For this review, take the finished solid that the model builds, in its own axes (mm). Face numbers are marked on the shaded views. Give positions to 0.01 mm unless a question says otherwise; leave off trailing zeros. Write each loop counter-clockwise with the first axis right and the second up, starting at its lowest first coordinate (ties: lowest second). Pieces come first, ordered by that corner, then holes.
Q1. We need section C-C (y = -45.5). Write out the cut boundary in (x, z), then the cut area to 3 significant figures.
Q2. We need section A-A (y = 6). Write out the cut boundary in (x, z).
Q3. We need section D-D (x = -46). Write out the cut boundary in (y, z), then the cut area to 3 significant figures.
Q4. Insertion check: P1, Ø1.5, axis at x = 0.5, y = -30, coming from the -Z side; P2, Ø12, axis at x = 58.5, y = -37.5, coming from the +Z side; P3, Ø4, axis at x = -30, y = 0, coming from the -Z side. Each pin has a flat end and moves straight along its axis. Give the tip position at first contact, or say it passes through.
Q5. Mouldability with a two-part tool opening along X and no side actions: class the marked faces 1, 2 and 3 as released by +X, released by -X, zero draft, split by the parting line, or undercut.
Q6. For line 1 (Y direction, x = 0, z = 0.5); line 2 (Z direction, x = -37.5, y = 56); line 3 (X direction, y = 0, z = -1.5), list the stretches that pass through material, from the lowest coordinate up.
Q7. We need section B-B (z = -4). Write out the cut boundary in (x, y), then the cut area to 3 significant figures.
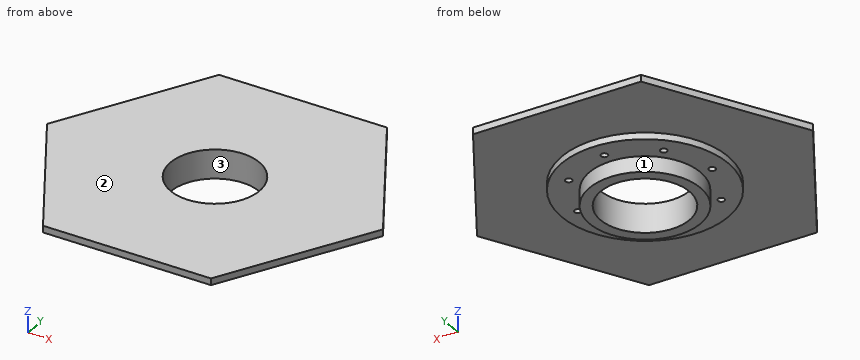
```python
from build123d import *

# Parameters (mm, degrees)
SKETCH_1_R               = 37.5
EXTRUDE_1_DEPTH          = 3
SKETCH_2_R               = 25
CUT_EXTRUDE_1_DEPTH      = 3
SKETCH_3_R               = 1.5
CUT_EXTRUDE_2_DEPTH      = 13
PATTERN_CIRCULAR_1_COUNT = 8
EXTRUDE_2_DEPTH          = 5
EXTRUDE_2_DEPTH_BACK     = 10
SKETCH_4_R               = 25
SKETCH_4_R_2             = 20
SKETCH_7_R               = 28.195307437
CUT_EXTRUDE_3_DEPTH      = 5
EXTRUDE_3_DEPTH          = 3
CUT_EXTRUDE_4_DEPTH      = 100.718353376
CUT_EXTRUDE_4_DEPTH_BACK = 100.718353376
SKETCH_9_R               = 20


with BuildPart() as part:
    # 草图1 → 凸台-拉伸1 (new body)
    with BuildSketch(Plane.XY):
        Circle(SKETCH_1_R)
    extrude(amount=EXTRUDE_1_DEPTH)

    # 草图2 → 切除-拉伸1 (cut)
    with BuildSketch(Plane(origin=(0, 0, 0), x_dir=(-1, 0, 0), z_dir=(0, 0, -1))):
        Circle(SKETCH_2_R)
    extrude(amount=-CUT_EXTRUDE_1_DEPTH, mode=Mode.SUBTRACT)

    # 草图3 → 切除-拉伸2 (cut)
    with BuildSketch(Plane.XY.offset(3)):
        with Locations((0, -30)):
            Circle(SKETCH_3_R)
    cut_extrude_2 = extrude(amount=-CUT_EXTRUDE_2_DEPTH, mode=Mode.SUBTRACT)

    # 阵列(圆周)1: 切除-拉伸2 ×8 about axis
    pattern_circular_1_axis = Axis((0, 0, 0), (0, 0, 1))
    for i in range(1, PATTERN_CIRCULAR_1_COUNT):
        add(cut_extrude_2.rotate(pattern_circular_1_axis, i * 360 / PATTERN_CIRCULAR_1_COUNT), mode=Mode.SUBTRACT)

    # 草图4 → 凸台-拉伸2 (add, two sides: drawn at the far end of the back side and taken through both)
    with BuildSketch(Plane.XY.offset(3).offset(-EXTRUDE_2_DEPTH_BACK)):
        with Locations(Location((0, 0, 0), (0, 0, 180))):
            Circle(SKETCH_4_R)
        Circle(SKETCH_4_R_2, mode=Mode.SUBTRACT)
    extrude(amount=EXTRUDE_2_DEPTH + EXTRUDE_2_DEPTH_BACK)

    # 草图7 → 切除-拉伸3 (cut)
    with BuildSketch(Plane.XY.offset(8)):
        Circle(SKETCH_7_R)
    extrude(amount=-CUT_EXTRUDE_3_DEPTH, mode=Mode.SUBTRACT)

    # 草图8 → 凸台-拉伸3 (add)
    with BuildSketch(Plane.XY.offset(3)):
        Polygon((37.5, 64.951905284), (-37.5, 64.951905284), (-75, 0), (-37.5, -64.951905284), (37.5, -64.951905284), (75, 0), align=None)
    extrude(amount=EXTRUDE_3_DEPTH)

    # 草图9 → 切除-拉伸4 (cut, two sides: drawn at the far end of the back side and taken through both)
    with BuildSketch(Plane(origin=(0, 0, 3), x_dir=(-1, 0, 0), z_dir=(0, 0, -1)).offset(-CUT_EXTRUDE_4_DEPTH_BACK)):
        Circle(SKETCH_9_R)
    extrude(amount=CUT_EXTRUDE_4_DEPTH + CUT_EXTRUDE_4_DEPTH_BACK, mode=Mode.SUBTRACT)


solid = part.part
```
Computed:
1. outline: (-48.73, 3) - (48.73, 3) - (48.73, 6) - (-48.73, 6) - close
1. area: 292 mm2
2. outline: (-71.54, 3) - (-37.02, 3) - (-37.02, 0) - (-24.27, 0) - (-24.27, -7) - (-19.08, -7) - (-19.08, 6) - (-71.54, 6) - close; (19.08, -7) - (24.27, -7) - (24.27, 0) - (37.02, 0) - (37.02, 3) - (71.54, 3) - (71.54, 6) - (19.08, 6) - close
3. outline: (-50.23, 3) - (50.23, 3) - (50.23, 6) - (-50.23, 6) - close
3. area: 301 mm2
4. P1: stops at z = 3
4. P2: stops at z = 6
4. P3: stops at z = 0
5. face 1: split by the parting line
5. face 2: zero draft
5. face 3: undercut
6. line 1: y = -37.5 to -31.5, -28.5 to -20, 20 to 28.5, 31.5 to 37.5
6. line 2: z = 3 to 6
6. line 3: x = -25 to -20, 20 to 25
7. outline: circle Ø50 at (0, 0); hole circle Ø40 at (0, 0)
7. area: 707 mm2
